```python
from build123d import *

# Parameters (mm, degrees)
SKETCH1_R           = 1
BOSS_EXTRUDE1_DEPTH = 3
BOSS_EXTRUDE2_DEPTH = 16
BOSS_EXTRUDE3_DEPTH = 2
SKETCH4_W           = 4.5
SKETCH4_H           = 6.5
BOSS_EXTRUDE4_DEPTH = 1.6
BOSS_EXTRUDE5_DEPTH = 10.1
CUT_EXTRUDE1_DEPTH  = 10.1
SKETCH8_W           = 13
SKETCH8_H           = 4
CUT_EXTRUDE2_DEPTH  = 5
SKETCH9_W           = 10
SKETCH9_H           = 5
CUT_EXTRUDE3_DEPTH  = 5


# Read off the part's stored shape, not the designer's step: Boss-Extrude2
with BuildPart() as part:
    # Sketch1 → Boss-Extrude1 (new body)
    with BuildSketch(Plane(origin=(0, 0, 0), x_dir=(1, 0, 0), z_dir=(0, 1, 0))):
        with BuildLine():
            Line((4.5, -16.7), (4.5, -10.2))
            Line((4.5, -10.2), (25.5, -10.2))
            Line((25.5, -10.2), (25.5, 13.2))
            ThreePointArc((25.5, 13.2), (24.478451782, 14.991287847), (22.541960108, 15.7))
            Line((22.541960108, 15.7), (-19.05, 15.7))
            ThreePointArc((-19.05, 15.7), (-22.903731957, 14.103731957), (-24.5, 10.25))
            Line((-24.5, 10.25), (-24.5, -13.7))
            ThreePointArc((-24.5, -13.7), (-23.621320344, -15.821320344), (-21.5, -16.7))
            Line((-21.5, -16.7), (4.5, -16.7))
        make_face()
        with Locations(Location((23, 13.2, 0), (0, 0, 270))):
            Circle(SKETCH1_R, mode=Mode.SUBTRACT)
        with Locations(Location((-22, -14.2, 0), (0, 0, 270))):
            Circle(SKETCH1_R, mode=Mode.SUBTRACT)
    extrude(amount=BOSS_EXTRUDE1_DEPTH)

    # Boss-Extrude2 outline → Boss-Extrude2 (add)
    with BuildSketch(Plane(origin=(0, 3, 0), x_dir=(1, 0, 0), z_dir=(0, 1, 0))):
        with BuildLine():
            Line((-24.5, 10.25), (-24.5, -9.2))
            add(Edge.make_bspline(
                [(-24.5, -9.2), (-23.769282577, -14.160806345), (-16.834317029, -8.300272079), (-21.009947693, -15.748034375), (-17, -16.7)],
                knots=[0, 0, 0, 0, 0, 1, 1, 1, 1, 1], degree=4))
            Line((-17, -16.7), (4.5, -16.7))
            Line((4.5, -16.7), (4.5, -10.2))
            Line((4.5, -10.2), (25.5, -10.2))
            Line((25.5, -10.2), (25.5, 8.2))
            add(Edge.make_bspline(
                [(25.5, 8.2), (24.79086606, 13.172227374), (17.855900512, 7.311693108), (22.031531177, 14.759455405), (18, 15.7)],
                knots=[0, 0, 0, 0, 0, 1, 1, 1, 1, 1], degree=4))
            Line((18, 15.7), (-19.05, 15.7))
            ThreePointArc((-19.05, 15.7), (-22.903731957, 14.103731957), (-24.5, 10.25))
        make_face()
    extrude(amount=BOSS_EXTRUDE2_DEPTH)

    # Sketch3 → Boss-Extrude3 (add)
    with BuildSketch(Plane(origin=(0, 19, 0), x_dir=(1, 0, 0), z_dir=(0, 1, 0))):
        with BuildLine():
            Line((25.5, -10.2), (25.5, 8.2))
            add(Edge.make_bspline(
                [(25.5, 8.2), (24.79086606, 13.172227374), (17.855900512, 7.311693108), (22.031531177, 14.759455405), (18, 15.7)],
                knots=[0, 0, 0, 0, 0, 1, 1, 1, 1, 1], degree=4))
            Line((18, 15.7), (0, 15.7))
            Line((0, 15.7), (0, -10.2))
            Line((0, -10.2), (25.5, -10.2))
        make_face()
    extrude(amount=BOSS_EXTRUDE3_DEPTH)

    # Sketch4 → Boss-Extrude4 (add)
    with BuildSketch(Plane(origin=(0, 19, 0), x_dir=(1, 0, 0), z_dir=(0, 1, 0))):
        with Locations((2.25, -13.45)):
            Rectangle(SKETCH4_W, SKETCH4_H)
    extrude(amount=BOSS_EXTRUDE4_DEPTH)

    # Sketch5 → Boss-Extrude5 (add)
    with BuildSketch(Plane.XY.offset(10.2)):
        with BuildLine():
            Line((6, 0.5), (24, 0.5))
            ThreePointArc((24, 0.5), (24.707106781, 0.792893219), (25, 1.5))
            Line((25, 1.5), (25, 19.5))
            ThreePointArc((25, 19.5), (24.707106781, 20.207106781), (24, 20.5))
            Line((24, 20.5), (6, 20.5))
            ThreePointArc((6, 20.5), (5.292893219, 20.207106781), (5, 19.5))
            Line((5, 19.5), (5, 1.5))
            ThreePointArc((5, 1.5), (5.292893219, 0.792893219), (6, 0.5))
        make_face()
    extrude(amount=BOSS_EXTRUDE5_DEPTH)

    # Sketch7 → Cut-Extrude1 (cut)
    with BuildSketch(Plane.XY.offset(20.3)):
        with BuildLine():
            Line((14.357886119, 1.053511456), (14.357886119, 3.813652456))
            ThreePointArc((14.357886119, 3.813652456), (9.574356132, 7.008298347), (8.98130736, 12.729855361))
            Line((8.98130736, 12.729855361), (6.540165326, 14.017955408))
            ThreePointArc((6.540165326, 14.017955408), (7.229438492, 5.594282327), (14.357886119, 1.053511456))
        make_face()
        with BuildLine():
            Line((7.140555489, 15.255205238), (9.581697527, 13.967105189))
            ThreePointArc((9.581697527, 13.967105189), (15.216789935, 17.241147229), (20.990144219, 14.217573506))
            Line((20.990144219, 14.217573506), (23.405000511, 15.560138833))
            ThreePointArc((23.405000511, 15.560138833), (15.186710134, 19.998330789), (7.140555489, 15.255205238))
        make_face()
        with BuildLine():
            Line((24.047997852, 14.353815082), (21.559268085, 13.160247955))
            ThreePointArc((21.559268085, 13.160247955), (21.07012739, 6.908676596), (15.644806916, 3.764268729))
            Line((15.644806916, 3.764268729), (15.644806916, 1.004127729))
            ThreePointArc((15.644806916, 1.004127729), (23.404589952, 5.439208876), (24.047997852, 14.353815082))
        make_face()
    extrude(amount=-CUT_EXTRUDE1_DEPTH, mode=Mode.SUBTRACT)

    # Sketch8 → Cut-Extrude2 (cut)
    with BuildSketch(Plane(origin=(0, 19, 0), x_dir=(1, 0, 0), z_dir=(0, 1, 0))):
        with Locations((-9.95, 10.25)):
            Rectangle(SKETCH8_W, SKETCH8_H)
    extrude(amount=-CUT_EXTRUDE2_DEPTH, mode=Mode.SUBTRACT)

    # Sketch9 → Cut-Extrude3 (cut)
    with BuildSketch(Plane(origin=(0, 0, -15.7), x_dir=(-1, 0, 0), z_dir=(0, 0, -1))):
        with Locations((-8.95, 16.35)):
            Rectangle(SKETCH9_W, SKETCH9_H)
    extrude(amount=-CUT_EXTRUDE3_DEPTH, mode=Mode.SUBTRACT)


solid = part.part
```
Here's how the part is built. I have some questions about the finished solid (model axes, mm). A direction names the side the tool comes from. Round coordinates to 2 decimals unless told otherwise and drop trailing zeros. Loops run counter-clockwise (first coordinate to the right, second up) from the corner with the lowest first, then second, coordinate; pieces in that order, holes last. Notation, with made-up numbers: (-6, 15) -> (33, 15) arc R27 ccw to (33, 43) -> close; hole circle Ø10 at (-22, 86.25). An arc over 180 degrees is marked (long way). Answer as CSV lines item,"result". Start each with the question number.
1. I'm going to push flat-ended pins straight in: P1, Ø3, axis at y = 18, z = 16.5, coming from the +X side; P2, Ø3, axis at x = 17.5, z = 13, coming from the +Y side; P3, Ø3, axis at y = 2, z = 16, coming from the -X side; P4, Ø3, axis at x = 4, z = -6.5, coming from the -Y side. Where does each tip first touch, or does it pass through?
2. If we mould it in two halves opening along X, with no side actions, what happens to faces 6 (the face through (-20.7, 3, 14.3)), 7 (the face through (21.12, 6.99, 15.32)), 8 (the face through (24.715, 20.199, 15.179))? For each: pulls with the +X half, pulls with the -X half, needs draft (parallel to the pull), parting line crosses it, or undercut.
3. I need wall thicknesses on probe 1 along Z at (x, y) = (-11.5, 14.25); probe 2 along X at (y, z) = (0.7, 14.2); probe 3 along Y at (x, z) = (21, 16.5). Which ranges of each line are inside material? Lowest first, please. Write a range as from..to.
4. Imagine slicing it at B-B on z = 1.5. Write out the boundary of the cut face in (x, y).
5. Imagine slicing it at A-A on y = 2.25. Write out the boundary of the cut face in (x, z).
6. For faces 1 (the face through (-10, 17, -12.25)), 2 (the face through (3.95, 16, -13)), 3 (the face through (25, 12, 15)), 4 (the face through (-12, 19, 0)), 5 (the face through (14.358, 2, 15)), which set-ups out of +Z, -Z, +X, -X, +Y, -Y let a thin tool reach every point of the face, with its end or its side?
Solution:
1,P1,"x = 25"
1,P2,"y = 20.5"
1,P3,"x = -24.39"
1,P4,"y = 0"
2,face 6,"needs draft"
2,face 7,"undercut"
2,face 8,"pulls with the +X half"
3,probe 1,"-15.7..-12.25, -8.25..16.7"
3,probe 2,"-24.46..-23, -21..4.5, 5.4..24.6"
3,probe 3,"0.5..2.85, 6.8..14.22, 18.15..20.5"
4,outline,"(-24.5, 0) -> (25.5, 0) -> (25.5, 21) -> (0, 21) -> (0, 19) -> (-24.5, 19) -> close"
5,outline,"(-24.5, -10.25) arc R5.45 ccw to (-19.05, -15.7) -> (22.54, -15.7) arc R3 ccw to (25.5, -13.2) -> (25.5, 10.2) -> (25, 10.2) -> (25, 20.3) -> (20.08, 20.3) -> (20.08, 10.2) -> (15.64, 10.2) -> (15.64, 20.3) -> (14.36, 20.3) -> (14.36, 10.2) -> (10.65, 10.2) -> (10.65, 20.3) -> (5, 20.3) -> (5, 10.2) -> (4.5, 10.2) -> (4.5, 16.7) -> (-21.5, 16.7) arc R3 ccw to (-24.5, 13.7) -> close; hole circle Ø2 at (-22, 14.2); hole circle Ø2 at (23, -13.2)"
6,face 1,"+Y"
6,face 2,"-Z"
6,face 3,"+Z, +X, +Y, -Y"
6,face 4,"+Z, -Z, -X, +Y"
6,face 5,"+Z"
